```python
from build123d import *

# Parameters (mm, degrees)
BOSS_EXTRUDE1_DEPTH = 42
CUT_EXTRUDE1_DEPTH  = 43
SKETCH2_W           = 22
SKETCH2_H           = 42
SKETCH2_W_2         = 21
SKETCH2_H_2         = 41
BOSS_EXTRUDE2_DEPTH = 15
SKETCH2_2_W         = 21
SKETCH2_2_H         = 41
BOSS_EXTRUDE3_DEPTH = 3


with BuildPart() as part:
    # Sketch1 → Boss-Extrude1 (new body)
    with BuildSketch(Plane.XY):
        with BuildLine():
            Line((-11, 0), (11, 0))
            Line((11, 0), (17.464466094, -6.464466094))
            ThreePointArc((17.464466094, -6.464466094), (18.548329851, -11.913417162), (13.928932188, -15))
            Line((13.928932188, -15), (-13.928932188, -15))
            ThreePointArc((-13.928932188, -15), (-18.548329851, -11.913417162), (-17.464466094, -6.464466094))
            Line((-17.464466094, -6.464466094), (-11, 0))
        make_face()
    extrude(amount=BOSS_EXTRUDE1_DEPTH)

    # Sketch3 → Cut-Extrude1 (cut, through all)
    with BuildSketch(Plane.XY.offset(42)):
        with BuildLine():
            Line((-13.928932188, -13.4), (13.928932188, -13.4))
            ThreePointArc((13.928932188, -13.4), (17.070122599, -11.30112367), (16.333095244, -7.595836944))
            Line((16.333095244, -7.595836944), (10.3372583, -1.6))
            Line((10.3372583, -1.6), (-10.3372583, -1.6))
            Line((-10.3372583, -1.6), (-16.333095244, -7.595836944))
            ThreePointArc((-16.333095244, -7.595836944), (-17.070122599, -11.30112367), (-13.928932188, -13.4))
        make_face()
    extrude(amount=-CUT_EXTRUDE1_DEPTH, mode=Mode.SUBTRACT)

    # Sketch2 → Boss-Extrude2 (add)
    with BuildSketch(Plane(origin=(0, 0, 0), x_dir=(1, 0, 0), z_dir=(0, 1, 0))):
        with Locations((0, -21)):
            Rectangle(SKETCH2_W, SKETCH2_H)
        with Locations((0, -21)):
            Rectangle(SKETCH2_W_2, SKETCH2_H_2, mode=Mode.SUBTRACT)
    extrude(amount=BOSS_EXTRUDE2_DEPTH)

    # Sketch2<2> → Boss-Extrude3 (add)
    with BuildSketch(Plane(origin=(0, 0, 0), x_dir=(1, 0, 0), z_dir=(0, 1, 0))):
        with Locations((0, -21)):
            Rectangle(SKETCH2_2_W, SKETCH2_2_H)
    extrude(amount=BOSS_EXTRUDE3_DEPTH)


solid = part.part
```
For this review, take the finished solid that the model builds, in its own axes (mm). A direction names the side the tool comes from. Coordinates: 2 decimals unless noted, no trailing zeros. Order: outer loops, then holes, each group sorted by start corner. A loop starts at its lowest first (then second) coordinate and runs counter-clockwise, first axis right, second up. Notation, with made-up numbers: (73.25, -9) - (77.25, -9) arc R6 cw to (77.25, 0) - close; hole circle Ø7 at (67.25, -39). An arc over 180 degrees is marked (long way). Answer as a JSON object with one key per item and string values. Group by question number.
1. The part is to be moulded in two halves that separate along Y. For faces 1 (the flat face through (0, -15, 21)), 2 (the flat face through (10.5, 9, 21)), 3 (the cylindrical face through (17.05, -11.35, 21.29)), say which applies: pulls with the +Y half, pulls with the -Y half, needs draft (parallel to the pull), parting line crosses it, or undercut.
2. We need section D-D on y = -11.75. State the section outline as (x, z) points, then the cut area to 3 significant figures.
3. Clearance check with flat-ended pins moving along their axes: P1, Ø1, axis at y = 2, z = 26.5, coming from the +X side; P2, Ø6.5, axis at x = -4, z = 22, coming from the +Y side; P3, Ø3, axis at y = 0.5, z = 12, coming from the -X side; P4, Ø1.5, axis at x = -12.5, y = 3.5, coming from the +Z side. State where each tip first meets the part, or that it passes through.
4. For faces 4 (the flat face through (0, 3, 21)), 5 (the cylindrical face through (-17.09, -11.25, 21.29)), 6 (the flat face through (-11, 7, 21)), list the 3-axis set-ups (+Z, -Z, +X, -X, +Y, -Y) from which the entire face can be reached by the end or side of a thin tool; tool diameter is ignored.
5. For probe 1 along Y at (x, z) = (-4.5, 5); probe 2 along Z at (x, y) = (8.5, 9.75); probe 3 along X at (y, z) = (9.5, 29), list the stretches that pass through material, from the lowest coordinate up.
6. We need section B-B on x = 3. State the section outline as (y, z) points.
7. We need section C-C on y = 9.5. State the section outline as (x, z) points.
8. We need section A-A on z = 37. State the section outline as (x, y) points.
Final values:
{
 "1": {"face 1": "pulls with the -Y half", "face 2": "needs draft", "face 3": "undercut"},
 "2": {"outline": "(-18.61, 0) - (-16.84, 0) - (-16.84, 42) - (-18.61, 42) - close; (16.84, 0) - (18.61, 0) - (18.61, 42) - (16.84, 42) - close", "area": "149 mm²"},
 "3": {"P1": "x = 11", "P2": "y = 3", "P3": "x = -12", "P4": "through"},
 "4": {"face 4": "+Y", "face 5": "+Z, -Z", "face 6": "+Z, -Z, -X, +Y"},
 "5": {"probe 1": "-15 to -13.4, -1.6 to 3", "probe 2": "0 to 0.5, 41.5 to 42", "probe 3": "-11 to -10.5, 10.5 to 11"},
 "6": {"outline": "(-15, 0) - (-13.4, 0) - (-13.4, 42) - (-15, 42) - close; (-1.6, 0) - (15, 0) - (15, 0.5) - (3, 0.5) - (3, 41.5) - (15, 41.5) - (15, 42) - (-1.6, 42) - close"},
 "7": {"outline": "(-11, 0) - (11, 0) - (11, 42) - (-11, 42) - close; hole (-10.5, 0.5) - (10.5, 0.5) - (10.5, 41.5) - (-10.5, 41.5) - close"},
 "8": {"outline": "(-17.46, -6.46) arc R5 ccw to (-13.93, -15) - (13.93, -15) arc R5 ccw to (17.46, -6.46) - (11, 0) - (11, 15) - (10.5, 15) - (10.5, 3) - (-10.5, 3) - (-10.5, 15) - (-11, 15) - (-11, 0) - close; hole (-16.33, -7.6) arc R3.4 ccw to (-13.93, -13.4) - (13.93, -13.4) arc R3.4 ccw to (16.33, -7.6) - (10.34, -1.6) - (-10.34, -1.6) - close"}
}
